from build123d import *

# Parameters (mm, degrees)
SKETCH1_R           = 12.7
BOSS_EXTRUDE1_DEPTH = 2.3114
BOSS_EXTRUDE1_DRAFT = -1
SKETCH7_R           = 12.7
SKETCH7_R_2         = 10.922
BOSS_EXTRUDE3_DEPTH = 6.35
BOSS_EXTRUDE3_DRAFT = -1
DRAFT1_ANGLE        = 10
FILLET2_R           = 0.381


with BuildPart() as part:
    # Sketch1 → Boss-Extrude1 (with draft: the straight prism first)
    with BuildSketch(Plane(origin=(0, 0, 0), x_dir=(1, 0, 0), z_dir=(0, 1, 0))):
        Circle(SKETCH1_R)
    extrude(amount=-BOSS_EXTRUDE1_DEPTH)
    # Boss-Extrude1: the draft: its side faces are tilted about the plane it starts from
    boss_extrude1_sides = [part.faces().sort_by_distance(p)[0] for p in [
        (-12.7, -1.1557, 0),
    ]]
    draft(boss_extrude1_sides, Plane(origin=(0, 0, 0), x_dir=(1, 0, 0), z_dir=(0, 1, 0)), BOSS_EXTRUDE1_DRAFT)


with BuildPart() as boss_extrude3_tool:
    # Sketch7 → Boss-Extrude3 (with draft: the straight prism first)
    with BuildSketch(Plane(origin=(0, 0, 0), x_dir=(1, 0, 0), z_dir=(0, 1, 0))):
        Circle(SKETCH7_R)
        Circle(SKETCH7_R_2, mode=Mode.SUBTRACT)
    extrude(amount=-BOSS_EXTRUDE3_DEPTH)
    # Boss-Extrude3: the draft: its side faces are tilted about the plane it starts from
    boss_extrude3_sides = [boss_extrude3_tool.faces().sort_by_distance(p)[0] for p in [
        (-12.7, -3.175, 0),
        (-10.922, -3.175, 0),
    ]]
    draft(boss_extrude3_sides, Plane(origin=(0, 0, 0), x_dir=(1, 0, 0), z_dir=(0, 1, 0)), BOSS_EXTRUDE3_DRAFT)


with BuildPart() as part_1:
    add(part.part)

    # Boss-Extrude3: add boss_extrude3_tool
    add(boss_extrude3_tool.part)

    # Draft1
    draft1_faces = [part_1.faces().sort_by_distance(p)[0] for p in [
        (-10.99759265, -4.3307, 0),
    ]]
    draft(draft1_faces, Plane(origin=(0, -2.3114, 0), x_dir=(0, 0, -1), z_dir=(0, -1, 0)), DRAFT1_ANGLE)

    # Fillet2
    fillet2_edges = [part_1.edges().sort_by_distance(p)[0] for p in [
        (-12.589160338, -6.35, 0),
        (-11.674459781, -6.35, 0),
    ]]
    fillet(fillet2_edges, radius=FILLET2_R)


solid = part_1.part
Verification items for the finished model (mm, model axes). Give positions to 0.01 mm unless a question says otherwise; leave off trailing zeros. Put each result on its own line as item: value. Start each with the question number.
1. Go/stop test with flat-tipped pins: pin 1 Ø1.5 at (y, z) = (-3, -3) entering from +X; pin 2 Ø2 at (x, z) = (-1, 3.5) entering from -Y; pin 3 Ø12 at (x, z) = (10, -2) entering from -Y; pin 4 Ø1.5 at (y, z) = (-1, 4) entering from -X. Record where each tip stops, or that it passes through.
2. Scan lines: line 1 along Y through (x, z) = (-6.25, 5.75); line 2 along X through (y, z) = (-6, 10.75); line 3 along Z through (x, y) = (5.5, -4). Record each from-to range of solid material in increasing order. Write a range as [from, to].
3. Draft check along X on faces 1 (the face through (12, -3, -4)), 2 (the face through (0, -2.311, 0)), 3 (the face through (0, 0, 0)), 4 (the face through (5.073, -2.492, 9.754)). Enter one of: +X half, -X half, draft (parallel to the pull), parting line (faces both ways), or undercut.
Answer list:
1. pin 1: x = 12.45
1. pin 2: y = -2.31
1. pin 3: y = -6.35
1. pin 4: x = -12.26
2. line 1: [-2.31, 0]
2. line 2: [-6.56, -4.39], [4.39, 6.56]
2. line 3: [-11.37, -9.83], [9.83, 11.37]
3. face 1: parting line
3. face 2: undercut
3. face 3: draft
3. face 4: undercut
